Part model, mm, in its own coordinate system. Face numbers are marked on the shaded views. Give positions to 0.01 mm unless a question says otherwise; leave off trailing zeros. Order: outer loops, then holes, each group sorted by start corner. A loop starts at its lowest first (then second) coordinate and runs counter-clockwise, first axis right, second up. Notation, with made-up numbers: (-7, 60.5) - (47, 60.5) arc R20 ccw to (47, 85.5) - close; hole circle Ø4 at (37, -30.5). An arc over 180 degrees is marked (long way). Use a Markdown table: item, result. Add a question column.
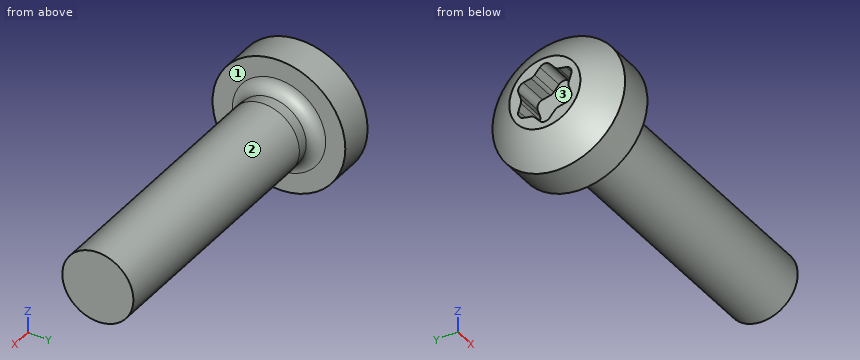
Autodesk Inventor part; units mm, degrees
ref_plane "YZ Plane" through (0, 0, 0) normal (1, 0, 0) x (0, 1, 0)
ref_plane "XZ Plane" through (0, 0, 0) normal (0, 1, 0) x (-1, 0, 0)
ref_plane "XY Plane" through (0, 0, 0) normal (0, 0, 1) x (1, 0, 0)
sketch "Sketch4" plane through (0, 0, 0) normal (0, 0, 1) x (1, 0, 0)
  line L0 (-2.4, 0) -> (12, 0)
  line L1 (0, 0) -> (-2.4, 0)
  line L2 (0, 2.8) -> (0, 1.97)
  line L3 (0.5, 1.47) -> (0.5, 1.47)
  line L4 (0.5, 1.47) -> (1, 1.5)
  arc A0 (0, 1.97) -> (0.5, 1.47) centre (0.5, 1.97) ccw
  line L5 (-2.4, 0) -> (-2.4, 1.5)
  line L6 (0, 2.8) -> (-1.4761, 2.8)
  arc A1 (-1.4761, 2.8) -> (-2.4, 1.5) centre (2.0854, -0.7093) ccw
  line L7 (1, 1.5) -> (12, 1.5)
  line L8 (12, 1.5) -> (12, 0)
  point P0 (0, 1.47)
  dimension "d71" = 0.5
  dimension "d72" = 12
  dimension "d74" = 0.5
  dimension "d75" = 2.94
  dimension "d78" = 3
  dimension "d82" = 5
  dimension "d83" = 2.4
  dimension "d84" = 5.6
  dimension "d104" = 11
  dimension "d105" = 3
revolve "Revolution7" add sketch "Sketch4" angle 360 about axis through (-2.4, 0, 0) along (1, 0, 0)
sketch "Sketch5" plane through (-2.4, 0, 0) normal (-1, 0, 0) x (0, 0, 1)
  circle A0 centre (0, 0) radius 1.4 construction
  circle A1 centre (0, 0) radius 0.98 construction
  line L0 (0, 0) -> (-0.8487, 0.49)
  line L1 (0, 0) -> (-0.8487, -0.49)
  line L2 (-1.8008, 0) -> (1.7887, 0)
  line L3 (-1.4, 0) -> (-0.8487, -0.49)
  line L4 (-1.4, 0) -> (-0.8487, 0.49)
  point P0 (0, 0)
  dimension "d88" = 2.8
  dimension "d89" = 1.96
  dimension "d90" = 30
  dimension "d91" = 30
extrude "Extrusion1" cut sketch "Sketch5" against normal blind 1.27
pattern_circular "Circular Pattern1" count 6 over 360 about axis through (-10, 0, 0) along (1, 0, 0) of "Extrusion1"
fillet "Fillet1" radius 0.28 12 edges at (-1.765, -1.2124, -0.7) (-1.765, -0.49, -0.8487) (-1.765, -0.98, 0) (-1.765, -1.2124, 0.7) (-1.765, -0.49, 0.8487) (-1.765, 0, 1.4) (-1.765, 0.98, 0) (-1.765, 1.2124, 0.7) (-1.765, 0.49, 0.8487) (-1.765, 0.49, -0.8487) (-1.765, 0, -1.4) (-1.765, 1.2124, -0.7)
thread "Thread7"
equation "\"a\" = 1"
equation "\"b\" = 11"
equation "\"dk\" = 5.6"
equation "\"k\" = 2.4"
equation "\"r\" = 0.5"
equation "\"rf\" = 5"
equation "\"x\" = 0.5"
equation "\"A_\" = 2.8"
equation "\"t\" = 1.27"
equation "\"p\" = 0.5"
equation "\"l_\" = 12"
equation "\"d\" = 3"
equation "\"ds_\" = 2.94"
equation "\"lg\" = 0"
properties part number "Flachkopfschraube mit Innenrund ISO 14583 - M3 x 12 - 4.8" material "Stahl"
1. Mould opens along Y. For the marked faces 1, 2 and 3 say: released by +Y, released by -Y, zero draft, split by the parting line, or undercut.
2. Drill centre lines: probe 1 along X at (y, z) = (0.35, -0.3); probe 2 along X at (y, z) = (1.75, -2.15); probe 3 along Y at (x, z) = (-1.5, -1.2). Where is each one in solid material? Low to high. Write a range as [from, to].
3. Pin check, flat tips, straight feed: P1, Ø1, axis at y = 0.5, z = 0.5, coming from the -X side; P2, Ø2, axis at x = 3, z = 2, coming from the +Y side; P3, Ø2, axis at x = 6, z = -0.5, coming from the -Y side. Stop position of each tip, or through.
4. Cut at B-B (x = -0.75). Write the cut outline in (y, z).
5. Cut at A-A (x = 4.25). Write the cut outline in (y, z).
Responses:
| question | item | result |
|---|---|---|
| 1 | face 1 | zero draft |
| 1 | face 2 | split by the parting line |
| 1 | face 3 | undercut |
| 2 | probe 1 | x = [-1.13, 12] |
| 2 | probe 2 | x = [-1.5, 0] |
| 2 | probe 3 | y = [-2.5, -0.17], [0.17, 2.5] |
| 3 | P1 | stops at x = -2.4 |
| 3 | P2 | stops at y = 1.12 |
| 3 | P3 | stops at y = -1.5 |
| 4 | outline | circle Ø5.6 at (0, 0) |
| 5 | outline | circle Ø3 at (0, 0) |
